Here's the drawing with two shaded views (mm, measured from the low corner). I have some questions. A direction names the side the tool comes from. Coordinates: 2 decimals unless noted, no trailing zeros. Loops run counter-clockwise (first coordinate to the right, second up) from the corner with the lowest first, then second, coordinate; pieces in that order, holes last.
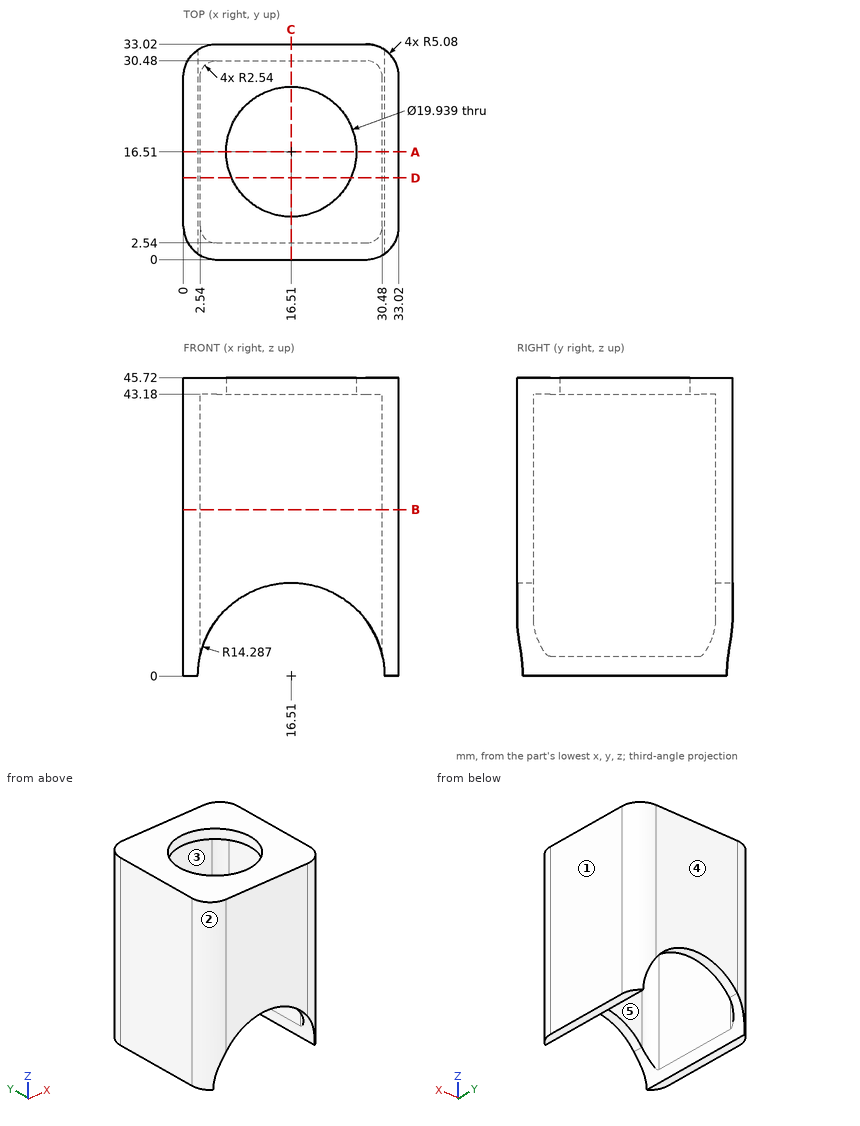
Q1. For the marked faces 4 and 5, which set-ups out of +Z, -Z, +X, -X, +Y, -Y let a thin tool reach every point of the face, with its end or its side?
Q2. Suppose I cut it at A-A on y = 16.51. Write out the boundary of the cut face in (x, z) (1 decimal).
Q3. Suppose I cut it at D-D on y = 12.5. Write out the boundary of the cut face in (x, z) (1 decimal).
Q4. Suppose I cut it at C-C on x = 16.51. Write out the boundary of the cut face in (y, z), and give its area (3 significant figures).
Q5. Please list where these lines run through material, in increasing order: probe 1 along Y at (x, z) = (22, 17.5); probe 2 along Y at (x, z) = (16, 44).
Q6. Will this pin go through, and if not, where does the flat tip stop? P1, Ø12, axis at x = 16.51, y = 16.51, coming from the +Z side.
Q7. Suppose I cut it at B-B on z = 25.5. Write out the boundary of the cut face in (x, y), and give its area (3 significant figures).
Q8. We'd pull the mould along Y, two halves only. Please class the marked faces 1, 2 and 3: pulls with the +Y half, pulls with the -Y half, needs draft (parallel to the pull), parting line crosses it, or undercut.
Check values:
1. face 4: +Z, -Z, +X, -X, +Y
1. face 5: -Z
2. outline: (0, 0) - (2.2, 0) arc R14.3 cw to (2.5, 3) - (2.5, 43.2) - (6.5, 43.2) - (6.5, 45.7) - (0, 45.7) - close; (26.5, 43.2) - (30.5, 43.2) - (30.5, 3) arc R14.3 cw to (30.8, 0) - (33, 0) - (33, 45.7) - (26.5, 45.7) - close
3. outline: (0, 0) - (2.2, 0) arc R14.3 cw to (2.5, 3) - (2.5, 43.2) - (7.4, 43.2) - (7.4, 45.7) - (0, 45.7) - close; (25.6, 43.2) - (30.5, 43.2) - (30.5, 3) arc R14.3 cw to (30.8, 0) - (33, 0) - (33, 45.7) - (25.6, 45.7) - close
4. outline: (0, 14.29) - (2.54, 14.29) - (2.54, 43.18) - (6.54, 43.18) - (6.54, 45.72) - (0, 45.72) - close; (26.48, 43.18) - (30.48, 43.18) - (30.48, 14.29) - (33.02, 14.29) - (33.02, 45.72) - (26.48, 45.72) - close
4. area: 180 mm2
5. probe 1: y = 0 to 2.54, 30.48 to 33.02
5. probe 2: y = 0 to 6.55, 26.47 to 33.02
6. P1: passes through
7. outline: (0, 5.08) arc R5.08 ccw to (5.08, 0) - (27.94, 0) arc R5.08 ccw to (33.02, 5.08) - (33.02, 27.94) arc R5.08 ccw to (27.94, 33.02) - (5.08, 33.02) arc R5.08 ccw to (0, 27.94) - close; hole (2.54, 5.08) arc R2.54 ccw to (5.08, 2.54) - (27.94, 2.54) arc R2.54 ccw to (30.48, 5.08) - (30.48, 27.94) arc R2.54 ccw to (27.94, 30.48) - (5.08, 30.48) arc R2.54 ccw to (2.54, 27.94) - close
7. area: 293 mm2
8. face 1: needs draft
8. face 2: pulls with the -Y half
8. face 3: undercut
